Geometry check sheet. Reference: the model listing, model coordinates, mm. Give positions to 0.01 mm unless a question says otherwise; leave off trailing zeros. Loops run counter-clockwise (first coordinate to the right, second up) from the corner with the lowest first, then second, coordinate; pieces in that order, holes last.
1. Cross-section at A-A, the plane z = 1361. Record the cut outline in (x, y), plus the area to 3 significant figures.
2. Go/stop test with flat-tipped pins: pin 1 Ø12.5 at (x, z) = (127, 12.7) entering from +Y; pin 2 Ø6.5 at (x, y) = (637.5, 3.5) entering from +Z. Record where each tip stops, or that it passes through.
3. Cross-section at B-B, the plane y = 3.75. State how many separate pieces and enclosed holes the cut face has, plus the area to 3 significant figures.
4. Material ranges on L1, parallel to Z at x = 1206.5, y = 3.5; L2, parallel to X at y = 4.25, z = 1574.8; L3, parallel to X at y = 6, z = 1117.6, recorded low to high.
5. Cross-section at C-C, the plane x = 407.5. Record the cut outline in (y, z).
from build123d import *

# Parameters (mm, degrees)
SKETCH1_W                              = 1219.2
SKETCH1_H                              = 12.7
BOSS_EXTRUDE1_DEPTH                    = 1828.8
SKETCH2_W                              = 660.4
SKETCH2_H                              = 508
CUT_EXTRUDE1_DEPTH                     = 13.7
F_3_8_0_375_DIAMETER_HOLE1_D           = 9.525
F_3_8_0_375_DIAMETER_HOLE1_CSINK_D     = 10.795
F_3_8_0_375_DIAMETER_HOLE1_CSINK_ANGLE = 90


with BuildPart() as part:
    # Sketch1 → Boss-Extrude1 (new body)
    with BuildSketch(Plane.XY):
        with Locations((609.6, 6.35)):
            Rectangle(SKETCH1_W, SKETCH1_H)
    extrude(amount=BOSS_EXTRUDE1_DEPTH)

    # Sketch2 → Cut-Extrude1 (cut, through all)
    with BuildSketch(Plane(origin=(0, 12.7, 0), x_dir=(1, 0, 0), z_dir=(0, 1, 0))):
        with Locations((609.6, -1574.8)):
            Rectangle(SKETCH2_W, SKETCH2_H)
    extrude(amount=-CUT_EXTRUDE1_DEPTH, mode=Mode.SUBTRACT)

    # 3/8 (0.375) Diameter Hole1 (through all)
    with Locations(Plane(origin=(0, 12.7, 0), x_dir=(1, 0, 0), z_dir=(0, 1, 0))):
        with Locations((1206.5, -1574.8), (1206.5, -1117.6), (1206.5, -660.4), (1206.5, -203.2), (12.7, -1574.8), (12.7, -1117.6), (12.7, -660.4), (12.7, -203.2), (444.5, -12.7), (127, -12.7), (1092.2, -12.7), (774.7, -12.7)):
            CounterSinkHole(F_3_8_0_375_DIAMETER_HOLE1_D / 2, F_3_8_0_375_DIAMETER_HOLE1_CSINK_D / 2, counter_sink_angle=F_3_8_0_375_DIAMETER_HOLE1_CSINK_ANGLE)


solid = part.part
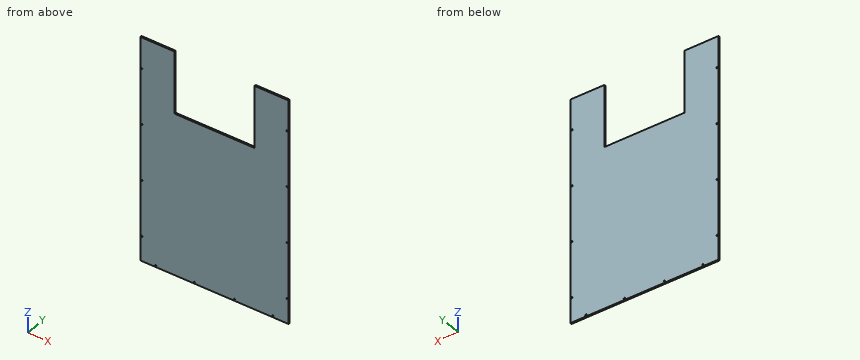
Result:
1. outline: (0, 0) - (279.4, 0) - (279.4, 12.7) - (0, 12.7) - close; (939.8, 0) - (1219.2, 0) - (1219.2, 12.7) - (939.8, 12.7) - close
1. area: 7,100 mm2
2. pin 1: stops at y = 12.7
2. pin 2: stops at z = 1320.8
3. separate pieces: 1
3. enclosed holes: 12
3. area: 1,890,000 mm2
4. L1: z = 0 to 198.44, 207.96 to 655.64, 665.16 to 1112.84, 1122.36 to 1570.04, 1579.56 to 1828.8
4. L2: x = 0 to 7.94, 17.46 to 279.4, 939.8 to 1201.74, 1211.26 to 1219.2
4. L3: x = 0 to 7.94, 17.46 to 1201.74, 1211.26 to 1219.2
5. outline: (0, 0) - (12.7, 0) - (12.7, 1320.8) - (0, 1320.8) - close
